Work out the finished part from the listing and answer in its coordinate system (mm). Face numbers are marked on the shaded views. A direction names the side the tool comes from. Give positions to 0.01 mm unless a question says otherwise; leave off trailing zeros. Loops run counter-clockwise (first coordinate to the right, second up) from the corner with the lowest first, then second, coordinate; pieces in that order, holes last.
from build123d import *

# Parameters (mm, degrees)
CORTAR_EXTRUIR1_START   = -10
CORTAR_EXTRUIR1_DEPTH   = 10
CROQUIS3_W              = 0.7
CROQUIS3_H              = 0.4
SALIENTE_EXTRUIR1_DEPTH = 3


with BuildPart() as part:
    # Croquis1 → Revolución1 (revolve)
    with BuildSketch(Plane.XY, mode=Mode.PRIVATE) as revoluci_n1_sk:
        with BuildLine():
            Line((0, 0), (0, 8.5))
            ThreePointArc((0, 8.5), (1.768113296, 7.629734533), (2.5, 5.8))
            Line((2.5, 5.8), (2.5, 0.8))
            Line((2.5, 0.8), (2.8, 0.8))
            Line((2.8, 0.8), (2.8, 0))
            Line((2.8, 0), (0, 0))
        make_face()
    revolve(revoluci_n1_sk.sketch.rotate(Axis((0, 0, 0), (0, 1, 0)), 90), axis=Axis((0, 0, 0), (0, 1, 0)))

    # Croquis2 → Cortar-Extruir1 (cut)
    with BuildSketch(Plane(origin=(0, 0.8, 0), x_dir=(1, 0, 0), z_dir=(0, 1, 0)).offset(CORTAR_EXTRUIR1_START)):
        with BuildLine():
            Line((-2.5, -1.260952021), (-2.5, 0))
            Line((-2.5, 0), (-2.8, 0))
            ThreePointArc((-2.8, 0), (-2.723967694, -0.64807407), (-2.5, -1.260952021))
        make_face()
        with BuildLine():
            Line((-2.8, 0), (-2.5, 0))
            Line((-2.5, 0), (-2.5, 1.260952021))
            ThreePointArc((-2.5, 1.260952021), (-2.723967694, 0.64807407), (-2.8, 0))
        make_face()
    extrude(amount=CORTAR_EXTRUIR1_DEPTH, mode=Mode.SUBTRACT)

    # Croquis3 → Saliente-Extruir1 (add)
    with BuildSketch(Plane.XZ):
        with Locations((-1.5, 0)):
            Rectangle(CROQUIS3_W, CROQUIS3_H)
        with Locations((1.5, 0)):
            Rectangle(CROQUIS3_W, CROQUIS3_H)
    extrude(amount=SALIENTE_EXTRUIR1_DEPTH)


solid = part.part
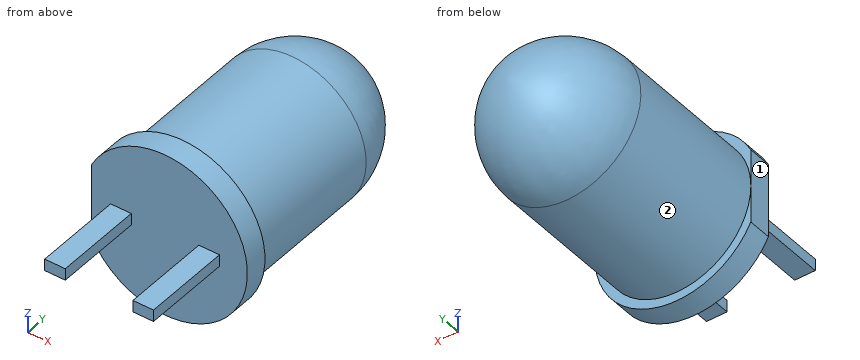
Item 1: Flat-ended cylindrical pins translate along their axes: pin 1 Ø0.8 at (x, y) = (1.5, -1) entering from +Z; pin 2 Ø3 at (y, z) = (3, 1.5) entering from +X; pin 3 Ø2 at (x, z) = (0, -0.5) entering from +Y; pin 4 Ø2 at (y, z) = (0, 2) entering from +X. Find the tip coordinate at first contact, or state that the pin passes through.
Item 2: Find section A-A, the plane y = -1.75. Write down the section's boundary in (x, z), plus the area to 3 significant figures.
Item 3: Consider line 1 (Y direction, x = -1.45, z = -2.1); line 2 (Z direction, x = 1.7, y = -1.5); line 3 (Y direction, x = -0.3, z = 0.35). Determine where each line is inside the solid, lowest interval first.
Item 4: For the marked faces 1 and 2, determine the directions among +Z, -Z, +X, -X, +Y, -Y from which every point of the face is accessible in a straight line to the end or side of a thin tool.
Item 5: Find section B-B, the plane y = 3. Write down the section's boundary in (x, z).
Ans:
1. pin 1: stops at z = 0.2
1. pin 2: stops at x = 2.5
1. pin 3: stops at y = 8.5
1. pin 4: stops at x = 2.62
2. outline: (-1.85, -0.2) - (-1.15, -0.2) - (-1.15, 0.2) - (-1.85, 0.2) - close; (1.15, -0.2) - (1.85, -0.2) - (1.85, 0.2) - (1.15, 0.2) - close
2. area: 0.560 mm2
3. line 1: y = 0 to 0.8
3. line 2: z = -0.2 to 0.2
3. line 3: y = 0 to 8.42
4. face 1: +Z, -Z, -X, +Y, -Y
4. face 2: +Y
5. outline: circle Ø5 at (0, 0)
